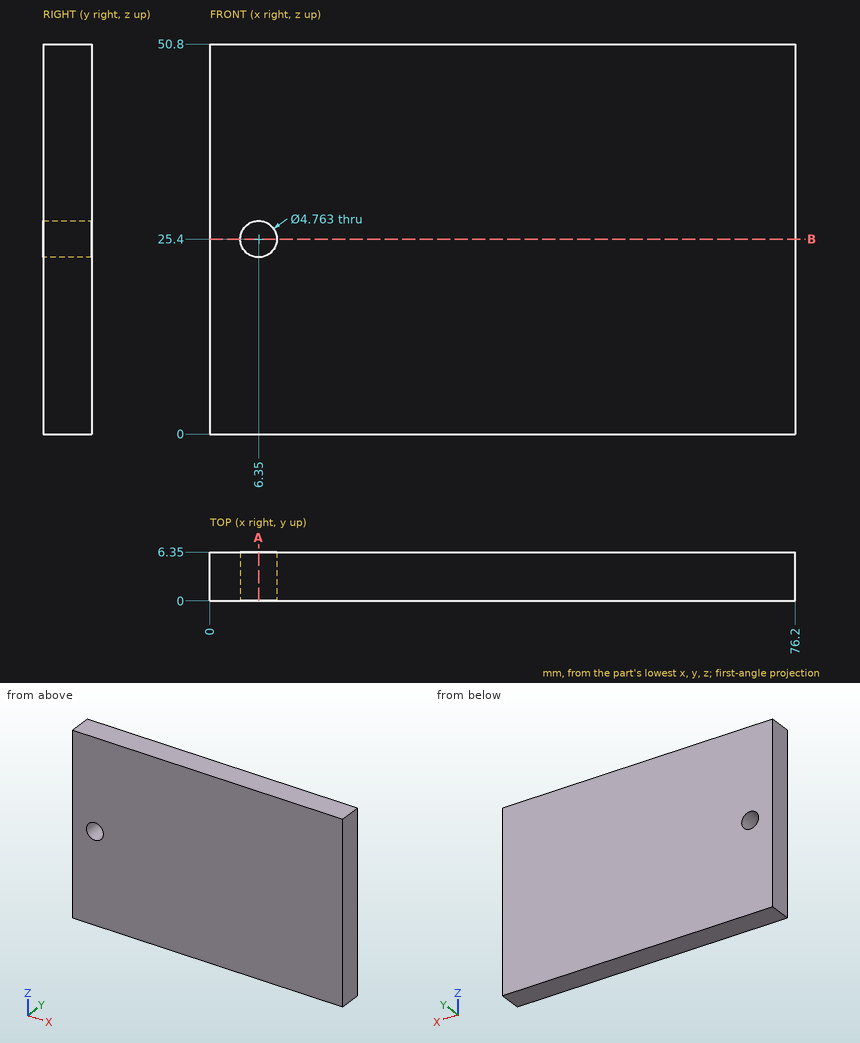
The drawing under review shows one solid part. Ordinate dimensions are in mm from its lowest x, y, z. Coordinates: 2 decimals unless noted, no trailing zeros. Order: outer loops, then holes, each group sorted by start corner. A loop starts at its lowest first (then second) coordinate and runs counter-clockwise, first axis right, second up. Notation, with made-up numbers: (65.25, 9.25) -> (102.25, 9.25) arc R18 cw to (102.25, 14.25) -> close; hole circle Ø8 at (68, 55). An arc over 180 degrees is marked (long way). Return JSON: item names as keys, results as strings.
1. We need section A-A on x = 6.35. Write out the cut boundary in (y, z).
Answer block:
{"outline": "(0, 0) -> (6.35, 0) -> (6.35, 23.02) -> (0, 23.02) -> close; (0, 27.78) -> (6.35, 27.78) -> (6.35, 50.8) -> (0, 50.8) -> close"}
2. We need section B-B on z = 25.4. Write out the cut boundary in (x, y).
Answer block:
{"outline": "(0, 0) -> (3.97, 0) -> (3.97, 6.35) -> (0, 6.35) -> close; (8.73, 0) -> (76.2, 0) -> (76.2, 6.35) -> (8.73, 6.35) -> close"}
3. For line 1 (X direction, y = 4.25, z = 25.4); line 2 (X direction, y = 2.5, z = 23.5) (1 decimal), list the stretches that pass through material, from the lowest coordinate up. Write a range as from..to.
Answer block:
{"line 1": "0..3.97, 8.73..76.2", "line 2": "0..4.9, 7.8..76.2"}
4. For pin 1 Ø12 at (x, z) = (18.5, 20) entering from -Y, flat-tipped, find the tip position at first contact; note if it passes through.
Answer block:
{"pin 1": "y = 0"}
